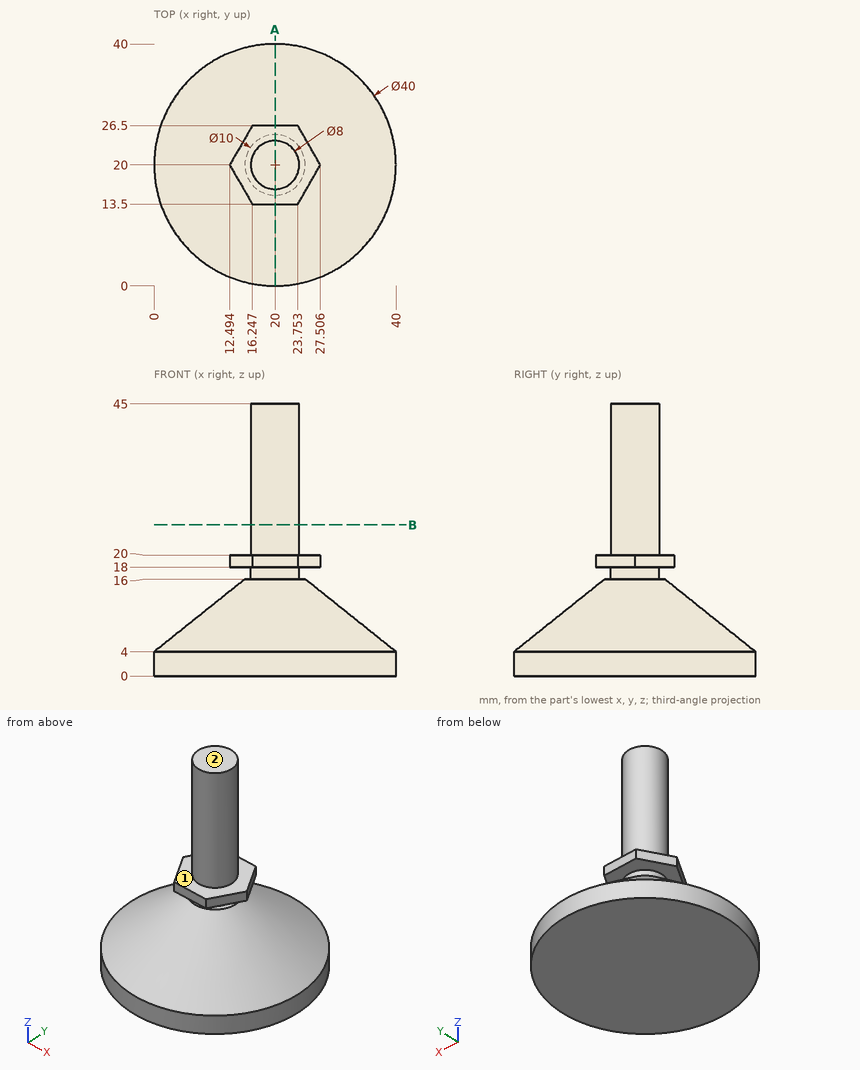
Geometry check sheet. Reference: drawing and pictorial views, mm from the part's lowest x, y, z. A direction names the side the tool comes from. Give positions to 0.01 mm unless a question says otherwise; leave off trailing zeros. Order: outer loops, then holes, each group sorted by start corner. A loop starts at its lowest first (then second) coordinate and runs counter-clockwise, first axis right, second up. Notation, with made-up numbers: M 38.5,37 L 83.5,37 A27 ccw 83.5,55 Z; hole C 8.5,65.5 d7. An arc over 180 degrees is marked long. Answer in a Markdown table with one row per item. Add a question column.
Item 1: Scan lines: probe 1 along Z at (x, y) = (9, 30.5) (1 decimal); probe 2 along Z at (x, y) = (30, 35); probe 3 along X at (y, z) = (16.5, 5.5) (1 decimal). Record each from-to range of solid material in increasing order. Write a range as from..to.
Item 2: Section check B-B, the plane z = 25. Enter the section's corners in (x, y).
Item 3: Tool access check on the marked faces 1 and 2. Record the directions out of +Z, -Z, +X, -X, +Y, -Y that give a thin tool (end or side, any length) a straight path to the whole face; none if there is none.
Item 4: Gauge pin test, flat ends, axial feed: pin 1 (2 mm diameter, centred on x = 20.5, z = 19, fed in from +Y); pin 2 (1 mm diameter, centred on x = 20.5, z = 18.5, fed in from -Y); pin 3 (3 mm diameter, centred on x = 21, z = 26, fed in from -Y). Record the tip position at first contact, or that the pin passes through.
Item 5: Section check A-A, the plane x = 20. Enter the section's corners in (y, z).
Filled sheet:
| question | item | result |
|---|---|---|
| 1 | probe 1 | z = 0..7.8 |
| 1 | probe 2 | z = 0..5.58 |
| 1 | probe 3 | x = 2.2..37.8 |
| 2 | outline | C 20,20 d8 |
| 3 | face 1 | +Z |
| 3 | face 2 | +Z, +X, -X, +Y, -Y |
| 4 | pin 1 | stops at y = 26.5 |
| 4 | pin 2 | stops at y = 13.5 |
| 4 | pin 3 | stops at y = 16 |
| 5 | outline | M 0,0 L 40,0 L 40,4 L 25,16 L 24,16 L 24,18 L 26.5,18 L 26.5,20 L 24,20 L 24,45 L 16,45 L 16,20 L 13.5,20 L 13.5,18 L 16,18 L 16,16 L 15,16 L 0,4 Z |
